Autodesk Fusion 360 part; units mm, degrees
sketch "Sketch1" plane through (0, 0, 0) normal (0, 0, 1) x (1, 0, 0)
  line L0 (0, 0) -> (100, 0)
  line L1 (0, 0) -> (0, 50)
  line L2 (0, 50) -> (100, 50)
  line L3 (100, 50) -> (100, 0)
  dimension "d1" = 100
  dimension "d2" = 50
extrude "Extrude1" add sketch "Sketch1" along normal blind 15
sketch "Sketch2" plane through (0, 0, 15) normal (0, 0, 1) x (-1, 0, 0)
  line L0 (0, 0) -> (-100, 0)
  line L1 (-100, 0) -> (-100, -50)
  line L2 (-100, -50) -> (0, -50)
  line L3 (0, -50) -> (0, 0)
  line L4 (-20, -50) -> (-35, 0)
  line L5 (-80, -50) -> (-65, 0)
  dimension "d6" = 35
  dimension "d7" = 20
  dimension "d8" = 35
  dimension "d9" = 20
extrude "Extrude2" add sketch "Sketch2" along normal blind 35 contours L0 L2 L3 L4
extrude "Extrude3" add sketch "Sketch2" along normal blind 35 contours L0 L1 L2 L5
chamfer "Chamfer1" distance 50 distance2 35 1 edges at (17.5, 0, 50) measured on face at (18.3333, 16.6667, 50)
chamfer "Chamfer1" distance 50 distance2 35 1 edges at (82.5, 0, 50) measured on face at (81.6667, 16.6667, 50)
The listing builds one solid part. Answer for the finished solid, in the listing's coordinates (mm). A direction names the side the tool comes from. Give positions to 0.01 mm unless a question says otherwise; leave off trailing zeros. Write each loop counter-clockwise with the first axis right and the second up, starting at its lowest first coordinate (ties: lowest second). Pieces come first, ordered by that corner, then holes. Notation, with made-up numbers: (55, -5.5) - (69, -5.5) arc R9 ccw to (69, 7.5) - close; hole circle Ø8 at (32.25, -19.5). An arc over 180 degrees is marked (long way). Use a Markdown table: item, result.
1. Section D-D on z = 41.5 is taken. Write down the section's boundary in (x, y).
Values follow:
| item | result |
|---|---|
| outline | (0, 37.85) - (23.65, 37.85) - (20, 50) - (0, 50) - close; (76.35, 37.85) - (100, 37.85) - (100, 50) - (80, 50) - close |
2. A tool of negligible diameter and unlimited length cuts with its end or side. For faces 5 (the flat face through (51, 50, 14)), 6 (the flat face through (50, 31, 15)), from which of +Z, -Z, +X, -X, +Y, -Y can it reach the whole face along a straight path? Write none if from no direction.
Values follow:
| item | result |
|---|---|
| face 5 | +Z, -Z, +X, -X, +Y |
| face 6 | +Z, +Y |
3. Find the intervals of material crossed by probe 1 along Z at (x, y) = (48, 36); probe 2 along X at (y, z) = (41, 38.5); probe 3 along Y at (x, z) = (88.5, 26), in increasing order. Write a range as from..to.
Values follow:
| item | result |
|---|---|
| probe 1 | z = 0..15 |
| probe 2 | x = 0..22.7, 77.3..100 |
| probe 3 | y = 15.7..50 |
4. For a pull along X with two mould halves and no side action, classify faces 1 (the flat face through (0, 30, 19)), 2 (the flat face through (13.37, 24.65, 32.26)), 3 (the flat face through (74.272, 30.906, 28.366)), 4 (the flat face through (25.728, 30.906, 28.366)) as released by +X, released by -X, zero draft, split by the parting line, or undercut.
Values follow:
| item | result |
|---|---|
| face 1 | released by -X |
| face 2 | zero draft |
| face 3 | undercut |
| face 4 | undercut |
5. Each of these flat-tipped pins is pushed along its axis until it touches: P1, Ø2, axis at x = 81, y = 30, coming from the +Z side; P2, Ø1, axis at x = 67.5, y = 15, coming from the +Z side; P3, Ø12, axis at x = 11.5, z = 42.5, coming from the -Y side; P4, Ø3, axis at x = 71.5, z = 38.5, coming from the +Y side. Where does it stop, or does it pass through?
Values follow:
| item | result |
|---|---|
| P1 | stops at z = 36.71 |
| P2 | stops at z = 15 |
| P3 | stops at y = 30.7 |
| P4 | passes through |
6. Section A-A on z = 31 is taken. Write down the section's boundary in (x, y).
Values follow:
| item | result |
|---|---|
| outline | (0, 22.85) - (28.15, 22.85) - (20, 50) - (0, 50) - close; (71.85, 22.85) - (100, 22.85) - (100, 50) - (80, 50) - close |
7. Section B-B on y = 39 is taken. Write down the section's boundary in (x, z).
Values follow:
| item | result |
|---|---|
| outline | (0, 0) - (100, 0) - (100, 42.31) - (76.7, 42.31) - (76.7, 15) - (23.3, 15) - (23.3, 42.31) - (0, 42.31) - close |
